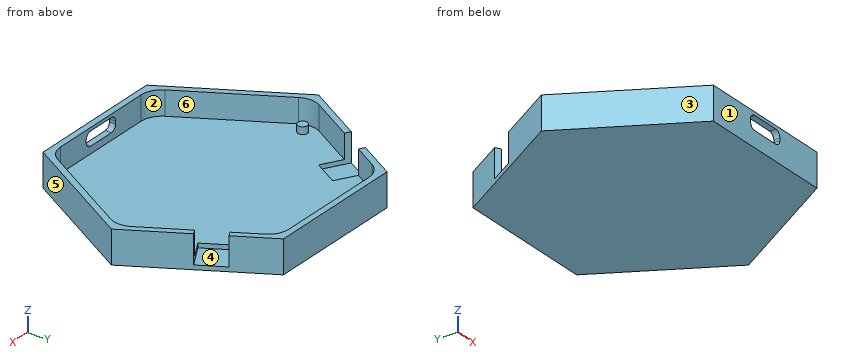
from build123d import *

# Parameters (mm, degrees)
PAD_DEPTH          = 2
PAD001_DEPTH       = 5.5
POCKET_DEPTH       = 6.5
POCKET001_DEPTH    = 5
SKETCH004_R        = 1.1
PAD002_DEPTH       = 1.6
POLARPATTERN_COUNT = 4
POLARPATTERN_ANGLE = 180


with BuildPart() as part:
    # Sketch → Pad (new body)
    with BuildSketch(Plane.XY):
        Polygon((-31.6, 0), (-15.8, -27.366403), (15.8, -27.366403), (31.6, 0), (15.8, 27.366403), (-15.8, 27.366403), align=None)
    extrude(amount=PAD_DEPTH)

    # Sketch001 (on Face8 of Pad) → Pad001 (join)
    with BuildSketch(Plane.XY.offset(2)):
        Polygon((-31.6, 0), (-15.8, -27.366403), (15.8, -27.366403), (31.6, 0), (15.8, 27.366403), (-15.8, 27.366403), align=None)
        with BuildLine():
            Line((-28.65, -2.338268), (-16.365, -23.616513))
            ThreePointArc((-16.365, -23.616513), (-14.634249, -25.347263), (-12.27, -25.980762))
            Line((-12.27, -25.980762), (12.273, -25.980762))
            ThreePointArc((12.273, -25.980762), (14.634651, -25.34796), (16.3635, -23.619111))
            Line((16.3635, -23.619111), (28.63635, -2.361911))
            ThreePointArc((28.63635, -2.361911), (29.269222, 0), (28.63635, 2.361911))
            Line((28.63635, 2.361911), (16.35, 23.642494))
            ThreePointArc((16.35, 23.642494), (14.638269, 25.354225), (12.3, 25.980762))
            Line((12.3, 25.980762), (-12, 25.980762))
            ThreePointArc((-12, 25.980762), (-14.598076, 25.28461), (-16.5, 23.382686))
            Line((-16.5, 23.382686), (-28.65, 2.338269))
            ThreePointArc((-28.65, 2.338269), (-29.276537, 0), (-28.65, -2.338268))
        make_face(mode=Mode.SUBTRACT)
    extrude(amount=PAD001_DEPTH)

    # Sketch002 (on Face11 of Pad001) → Pocket (cut)
    with BuildSketch(Plane.XY.offset(7.5)):
        Polygon((-24.04408, 13.087238), (-20.79408, 18.716403), (-15.164915, 15.466403), (-18.414915, 9.837238), align=None)
        Polygon((20.79408, 18.716403), (24.04408, 13.087238), (18.414915, 9.837238), (15.164915, 15.466403), align=None)
    extrude(amount=-POCKET_DEPTH, mode=Mode.SUBTRACT)

    # Sketch003 (on Face13 of Pocket) → Pocket001 (cut)
    with BuildSketch(Plane.XZ.offset(27.366403)):
        with BuildLine():
            Line((-3.175, 6.76), (3.175, 6.76))
            ThreePointArc((4.475, 5.46), (4.094239, 6.379239), (3.175, 6.76))
            Line((4.475, 5.46), (4.475, 4.9))
            ThreePointArc((3.175, 3.6), (4.094239, 3.980761), (4.475, 4.9))
            Line((3.175, 3.6), (-3.175, 3.6))
            ThreePointArc((-4.475, 4.9), (-4.094239, 3.980761), (-3.175, 3.6))
            Line((-4.475, 5.46), (-4.475, 4.9))
            ThreePointArc((-3.175, 6.76), (-4.094239, 6.379239), (-4.475, 5.46))
        make_face()
    extrude(amount=-POCKET001_DEPTH, mode=Mode.SUBTRACT)

    # Sketch004 (on Face16 of Pocket001) → Pad002 (join)
    with BuildSketch(Plane.XY.offset(2)):
        with Locations((-26.75, 0)):
            Circle(SKETCH004_R)
    pad002 = extrude(amount=PAD002_DEPTH)

    # PolarPattern: Pad002 ×4 about axis
    polarpattern_axis = Axis((0, 0, 2), (0, 0, -1))
    for i in range(1, POLARPATTERN_COUNT):
        add(pad002.rotate(polarpattern_axis, i * POLARPATTERN_ANGLE / (POLARPATTERN_COUNT - 1)))


solid = part.part
Here's how the part is built. I have some questions about the finished solid (model axes, mm). Face numbers are marked on the shaded views. A direction names the side the tool comes from. Give positions to 0.01 mm unless a question says otherwise; leave off trailing zeros. Order: outer loops, then holes, each group sorted by start corner. A loop starts at its lowest first (then second) coordinate and runs counter-clockwise, first axis right, second up. Notation, with made-up numbers: M -13.5,51.25 L 0.5,51.25 A26 cw 0.5,65.25 Z; hole C 20,-10.75 d6. An arc over 180 degrees is marked long. Answer as a JSON object with one key per item and string values. Group by question number.
1) I'm going to push flat-ended pins straight in: pin 1 Ø1.5 at (y, z) = (7.5, 6) entering from -X; pin 2 Ø8 at (x, y) = (23, 12) entering from +Z; pin 3 Ø1.5 at (y, z) = (-11, 5) entering from +X; pin 4 Ø3 at (y, z) = (10.5, 6.5) entering from +X. Where does each tip first touch, or does it pass through?
2) Suppose I cut it at D-D, the plane y = 20.5. Write out the boundary of the cut face in (x, z), plus the area to 3 significant figures.
3) We'd pull the mould along X, two halves only. Please class the marked faces 3, 4, 5 and 6: pulls with the +X half, pulls with the -X half, needs draft (parallel to the pull), parting line crosses it, or undercut.
4) Suppose I cut it at B-B, the plane y = 7.5. Write out the boundary of the cut face in (x, z).
5) Suppose I cut it at A-A, the plane x = 0.5. Write out the boundary of the cut face in (y, z), plus the area to 3 significant figures.
6) Please list where these lines run through material, in increasing order: L1, parallel to Y at x = 6.5, z = 7; L2, parallel to Z at x = -5.5, y = -21; L3, parallel to X at y = 9, z = 4. Write a range as [from, to].
7) Suppose I cut it at C-C, the plane x = 26.75. Write out the boundary of the cut face in (y, z).
8) On a 3-axis mill with a long thin cutter (end or side, diameter ignored), from which of +Z, -Z, +X, -X, +Y, -Y can I reach the whole of each face in a straight line? I mean the marked faces 1 and 2. Say none if no direction works.
Results found:
{
 "1": {"pin 1": "x = -27.7", "pin 2": "z = 7.5", "pin 3": "x = 25.68", "pin 4": "x = 26.4"},
 "2": {"outline": "M -19.76,0 L 19.76,0 L 19.76,7.5 L 18.16,7.5 L 18.16,2 L -18.16,2 L -18.16,7.5 L -19.76,7.5 Z", "area": "96.7 mm²"},
 "3": {"face 3": "pulls with the -X half", "face 4": "undercut", "face 5": "pulls with the +X half", "face 6": "undercut"},
 "4": {"outline": "M -27.27,0 L 27.27,0 L 27.27,7.5 L 25.67,7.5 L 25.67,2 L -25.67,2 L -25.67,7.5 L -27.27,7.5 Z"},
 "5": {"outline": "M -27.37,0 L 27.37,0 L 27.37,7.5 L 25.98,7.5 L 25.98,2 L -25.98,2 L -25.98,3.6 L -27.37,3.6 Z; M -27.37,6.76 L -25.98,6.76 L -25.98,7.5 L -27.37,7.5 Z", "area": "120 mm²"},
 "6": {"L1": "[-27.37, -25.98], [25.98, 27.37]", "L2": "[0, 2]", "L3": "[-26.4, -24.8], [24.8, 26.4]"},
 "7": {"outline": "M -8.4,0 L 8.4,0 L 8.4,7.5 L 5.63,7.5 L 5.63,2 L 1.1,2 L 1.1,3.6 L -1.1,3.6 L -1.1,2 L -5.63,2 L -5.63,7.5 L -8.4,7.5 Z"},
 "8": {"face 1": "+Z, -Z, +X, -X, -Y", "face 2": "+Z"}
}
